Check sheet for the modelled part. Datum: model origin and axes. Units: mm. A direction names the side the tool comes from. Round coordinates to 2 decimals unless told otherwise and drop trailing zeros. Loops run counter-clockwise (first coordinate to the right, second up) from the corner with the lowest first, then second, coordinate; pieces in that order, holes last. Notation, with made-up numbers: (37.5, 32.5) -> (43.5, 32.5) arc R32 ccw to (43.5, 68.5) -> close; hole circle Ø11 at (-4.75, -32.5). An arc over 180 degrees is marked (long way). Use one line per item in the form item = value. Start each with the question number.
(1) Set-up check for faces 1 (the flat face through (-128, -203.435, 18)), 2 (the flat face through (-43, -211, 0)): record each of +Z, -Z, +X, -X, +Y, -Y from which the full face is reachable in a straight line by a thin tool's end or side.
(2) Sectioned sample at A-A (z = 14). Record the cut outline in (x, y), and give its area (3 significant figures).
(3) Sectioned sample at B-B (x = -209.5). Record the cut outline in (y, z), and give its area (3 significant figures).
(4) Material ranges on probe 1 along Y at (x, z) = (-183, 32); probe 2 along X at (y, z) = (-94, 8), recorded low to high. Write a range as [from, to].
(5) Go/stop test with a flat-tipped pin: pin 1 (6 mm diameter, centred on x = -67.5, z = 18.5, fed in from +Y). Record where the tip stops, or that it passes through.
(6) Sectioned sample at C-C (y = -42). Record the cut outline in (x, z).
from build123d import *

# Parameters (mm, degrees)
F0_W     = 39.360307157
F0_H     = 36.9374714792
F1_DEPTH = 254
F2_W     = 50.564668417
F2_H     = 36.9374714792
F3_DEPTH = 259.6821213


# Not quite as in the source:
# - an extrude ends at something that could not be found from the text; its depth is read off the source's solid


with BuildPart() as f1:
    # F0 (on Front) → F1 (new body)
    with BuildSketch(Plane.XZ):
        with Locations((19.6801535785, 18.4687357396)):
            Rectangle(F0_W, F0_H)
    extrude(amount=F1_DEPTH)

    # F2 (on face) → F3 (join, through all)
    with BuildSketch(Plane(origin=(0, 0, 0), x_dir=(0, -1, 0), z_dir=(-1, 0, 0))):
        with Locations((228.7176657915, 18.4687357396)):
            Rectangle(F2_W, F2_H)
    extrude(amount=F3_DEPTH)


solid = f1.part
Checks:
q1.face_1 = +Z, -Z, -X, +Y
q1.face_2 = -Z, +X, -X, +Y, -Y
q2.outline = (-259.68, -254) -> (39.36, -254) -> (39.36, 0) -> (0, 0) -> (0, -203.44) -> (-259.68, -203.44) -> close
q2.area = 23,100 mm2
q3.outline = (-254, 0) -> (-203.44, 0) -> (-203.44, 36.94) -> (-254, 36.94) -> close
q3.area = 1,870 mm2
q4.probe_1 = [-254, -203.44]
q4.probe_2 = [0, 39.36]
q5.pin_1 = -203.44
q6.outline = (0, 0) -> (39.36, 0) -> (39.36, 36.94) -> (0, 36.94) -> close
